from build123d import *

# Parameters (mm, degrees)
SALIENTE_EXTRUIR1_DEPTH = 10
CORTAR_EXTRUIR2_DEPTH   = 2.5
CROQUIS3_R              = 4.5
SALIENTE_EXTRUIR2_DEPTH = 1.5
CROQUIS4_R              = 1.5
CORTAR_EXTRUIR3_DEPTH   = 58.982756057
CROQUIS5_R              = 6.2
CORTAR_EXTRUIR4_DEPTH   = 8


with BuildPart() as part:
    # Croquis1 → Saliente-Extruir1 (new body)
    with BuildSketch(Plane(origin=(0, 0, 0), x_dir=(-1, 0, 0), z_dir=(0, 0, -1))):
        with BuildLine():
            Line((-11.5, 55), (-4.5, 55))
            ThreePointArc((-4.5, 55), (-1.318019485, 53.681980515), (0, 50.5))
            Line((0, 50.5), (0, 10))
            ThreePointArc((0, 10), (-1.318019485, 6.818019485), (-4.5, 5.5))
            Line((-4.5, 5.5), (-11.5, 5.5))
            ThreePointArc((-11.5, 5.5), (-14.681980515, 6.818019485), (-16, 10))
            Line((-16, 10), (-16, 50.5))
            ThreePointArc((-16, 50.5), (-14.681980515, 53.681980515), (-11.5, 55))
        make_face()
    extrude(amount=-SALIENTE_EXTRUIR1_DEPTH)

    # Croquis2 → Cortar-Extruir2 (cut)
    with BuildSketch(Plane(origin=(0, 0, 0), x_dir=(-1, 0, 0), z_dir=(0, 0, -1))):
        Polygon((-8, 51.5), (-11.031088913, 49.75), (-11.031088913, 46.25), (-8, 44.5), (-4.968911087, 46.25), (-4.968911087, 49.75), align=None)
        Polygon((-8, 15.5), (-11.031088913, 13.75), (-11.031088913, 10.25), (-8, 8.5), (-4.968911087, 10.25), (-4.968911087, 13.75), align=None)
    extrude(amount=-CORTAR_EXTRUIR2_DEPTH, mode=Mode.SUBTRACT)

    # Croquis3 → Saliente-Extruir2 (add)
    with BuildSketch(Plane.XY.offset(10)):
        with Locations(Location((8, 48, 0), (0, 0, 180))):
            Circle(CROQUIS3_R)
        with Locations(Location((8, 12, 0), (0, 0, 180))):
            Circle(CROQUIS3_R)
    extrude(amount=SALIENTE_EXTRUIR2_DEPTH)

    # Croquis4 → Cortar-Extruir3 (cut, through all)
    with BuildSketch(Plane(origin=(0, 0, 2.5), x_dir=(-1, 0, 0), z_dir=(0, 0, -1))):
        with Locations((-8, 48)):
            Circle(CROQUIS4_R)
        with Locations((-8, 12)):
            Circle(CROQUIS4_R)
    extrude(amount=-CORTAR_EXTRUIR3_DEPTH, mode=Mode.SUBTRACT)

    # Croquis5 → Cortar-Extruir4 (cut)
    with BuildSketch(Plane.XY.offset(10)):
        with Locations((8, 30)):
            Circle(CROQUIS5_R)
    extrude(amount=-CORTAR_EXTRUIR4_DEPTH, mode=Mode.SUBTRACT)


solid = part.part
The model under review builds one solid part; all positions refer to its coordinate system, in mm. A direction names the side the tool comes from. Round coordinates to 2 decimals unless told otherwise and drop trailing zeros. Loops run counter-clockwise (first coordinate to the right, second up) from the corner with the lowest first, then second, coordinate; pieces in that order, holes last. Notation, with made-up numbers: (54, -5.5) - (61, -5.5) arc R27 cw to (61, 13.5) - close; hole circle Ø2 at (-12.5, -12). An arc over 180 degrees is marked (long way). Use CSV: the item, a comma, the result in double quotes.
(1) For line 1 (Y direction, x = 8, z = 5); line 2 (Z direction, x = 14.5, y = 20.5); line 3 (Y direction, x = 3.5, z = 2.75), list the stretches that pass through material, from the lowest coordinate up.
Working result:
line 1,"y = 5.5 to 10.5, 13.5 to 23.8, 36.2 to 46.5, 49.5 to 55"
line 2,"z = 0 to 10"
line 3,"y = 5.61 to 25.74, 34.26 to 54.89"
(2) Take a section at C-C, the plane y = 30. Give the boundary of the cut face in (x, z).
Working result:
outline,"(0, 0) - (16, 0) - (16, 10) - (14.2, 10) - (14.2, 2) - (1.8, 2) - (1.8, 10) - (0, 10) - close"
(3) Clearance check with flat-ended pins moving along their axes: P1, Ø1.8, axis at x = 9.5, y = 49.5, coming from the -Z side; P2, Ø6, axis at x = 4.5, y = 27.5, coming from the +Z side; P3, Ø6, axis at x = 6, y = 28, coming from the +Z side. State where each tip first meets the part, or that it passes through.
Working result:
P1,"stops at z = 2.5"
P2,"stops at z = 10"
P3,"stops at z = 2"
(4) Take a section at A-A, the plane z = 7. Give the boundary of the cut face in (x, y).
Working result:
outline,"(0, 10) arc R4.5 ccw to (4.5, 5.5) - (11.5, 5.5) arc R4.5 ccw to (16, 10) - (16, 50.5) arc R4.5 ccw to (11.5, 55) - (4.5, 55) arc R4.5 ccw to (0, 50.5) - close; hole circle Ø12.4 at (8, 30); hole circle Ø3 at (8, 12); hole circle Ø3 at (8, 48)"
(5) Take a section at D-D, the plane y = 47.5. Give the boundary of the cut face in (x, z), plus the area to 3 significant figures.
Working result:
outline,"(0, 0) - (4.97, 0) - (4.97, 2.5) - (6.59, 2.5) - (6.59, 11.5) - (3.53, 11.5) - (3.53, 10) - (0, 10) - close; (9.41, 2.5) - (11.03, 2.5) - (11.03, 0) - (16, 0) - (16, 10) - (12.47, 10) - (12.47, 11.5) - (9.41, 11.5) - close"
area,"133 mm^2"
(6) The part is to be moulded in two halves that separate along X. For faces 4 (the flat face through (8, 55, 5)), 5 (the cylindrical face through (1.283, 6.853, 4.93)), 6 (the flat face through (6.51, 9.36, 1.23)), say which applies: pulls with the +X half, pulls with the -X half, needs draft (parallel to the pull), parting line crosses it, or undercut.
Working result:
face 4,"needs draft"
face 5,"pulls with the -X half"
face 6,"undercut"
(7) Take a section at B-B, the plane y = 12. Give the boundary of the cut face in (x, z), plus the area to 3 significant figures.
Working result:
outline,"(0, 0) - (4.97, 0) - (4.97, 2.5) - (6.5, 2.5) - (6.5, 11.5) - (3.5, 11.5) - (3.5, 10) - (0, 10) - close; (9.5, 2.5) - (11.03, 2.5) - (11.03, 0) - (16, 0) - (16, 10) - (12.5, 10) - (12.5, 11.5) - (9.5, 11.5) - close"
area,"131 mm^2"
(8) Machinability: for faces 1 (the cylindrical face through (3.708, 10.648, 10.74)), 2 (the cylindrical face through (14.647, 6.783, 4.93)), 3 (the flat face through (4.969, 12, 1)), which of the approach directions +Z, -Z, +X, -X, +Y, -Y give a long, thin tool a straight path to every point of the face, cutting with its end or side? Answer none if there is none.
Working result:
face 1,"+Z"
face 2,"+Z, -Z, +X, -Y"
face 3,"-Z"
